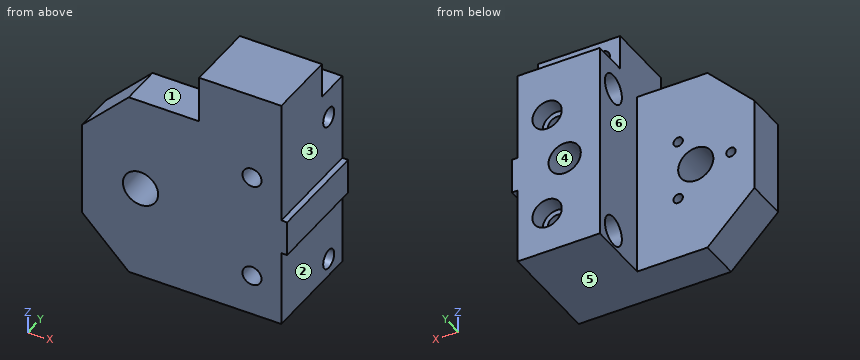
from build123d import *

# Parameters (mm, degrees)
BOSS_EXTRUDE1_DEPTH = 11.1125
BOSS_EXTRUDE2_START = -11.1125
SKETCH2_W           = 44.45
SKETCH2_H           = 127
BOSS_EXTRUDE2_DEPTH = 38.1
BOSS_EXTRUDE3_START = 26.9875
SKETCH3_W           = 44.45
SKETCH3_H           = 107.95
BOSS_EXTRUDE3_DEPTH = 19.05
BOSS_EXTRUDE4_START = -11.1125
SKETCH4_W           = 3.175
SKETCH4_H           = 19.0246
BOSS_EXTRUDE4_DEPTH = 57.15
CUT_EXTRUDE2_START  = 11.1125
SKETCH5_R           = 9.525
CUT_EXTRUDE2_DEPTH  = 131.386478852
CUT_EXTRUDE4_START  = 11.1125
SKETCH6_R           = 2.5527
CUT_EXTRUDE4_DEPTH  = 12.7
CUT_EXTRUDE6_START  = 11.1125
SKETCH7_R           = 2.5527
CUT_EXTRUDE6_DEPTH  = 12.7
CUT_EXTRUDE8_START  = 46.0375
SKETCH8_R           = 8.73125
CUT_EXTRUDE8_DEPTH  = 31.75
CUT_EXTRUDE10_START = 26.9875
SKETCH9_R           = 3.96875
CUT_EXTRUDE10_DEPTH = 19.05
CUT_EXTRUDE12_START = 46.0375
SKETCH10_R          = 5.1562
CUT_EXTRUDE12_DEPTH = 166.311478852
CUT_EXTRUDE14_START = 46.0375
SKETCH11_R          = 7.9375
CUT_EXTRUDE14_DEPTH = 9.525
CUT_EXTRUDE16_START = 31.75
SKETCH12_R          = 5.1562
CUT_EXTRUDE16_DEPTH = 88.523978852
CUT_EXTRUDE18_START = 31.75
SKETCH13_R          = 7.9375
CUT_EXTRUDE18_DEPTH = 9.525


with BuildPart() as part:
    # Sketch1 → Boss-Extrude1 (new, symmetric)
    with BuildSketch(Plane(origin=(0, 0, 0), x_dir=(1, 0, 0), z_dir=(0, 1, 0))):
        Polygon((-31.75, -25.4), (-6.35, -50.8), (31.75, -50.8), (31.75, 50.8), (-6.35, 50.8), (-31.75, 25.4), align=None)
    extrude(amount=BOSS_EXTRUDE1_DEPTH, both=True)

    # Sketch2 → Boss-Extrude2 (add)
    with BuildSketch(Plane(origin=(0, 0, 0), x_dir=(1, 0, 0), z_dir=(0, 1, 0)).offset(BOSS_EXTRUDE2_START)):
        with Locations((53.975, -12.7)):
            Rectangle(SKETCH2_W, SKETCH2_H)
    extrude(amount=BOSS_EXTRUDE2_DEPTH)

    # Sketch3 → Boss-Extrude3 (add)
    with BuildSketch(Plane(origin=(0, 0, 0), x_dir=(1, 0, 0), z_dir=(0, 1, 0)).offset(BOSS_EXTRUDE3_START)):
        with Locations((53.975, -3.175)):
            Rectangle(SKETCH3_W, SKETCH3_H)
    extrude(amount=BOSS_EXTRUDE3_DEPTH)

    # Sketch4 → Boss-Extrude4 (add)
    with BuildSketch(Plane(origin=(0, 0, 0), x_dir=(1, 0, 0), z_dir=(0, 1, 0)).offset(BOSS_EXTRUDE4_START)):
        with Locations((77.7875, 0.0127)):
            Rectangle(SKETCH4_W, SKETCH4_H)
    extrude(amount=BOSS_EXTRUDE4_DEPTH)

    # Sketch5 → Cut-Extrude2 (cut, through all)
    with BuildSketch(Plane(origin=(0, 0, 0), x_dir=(1, 0, 0), z_dir=(0, 1, 0)).offset(CUT_EXTRUDE2_START)):
        with Locations(Location((0, 0, 0), (0, 0, 270))):
            Circle(SKETCH5_R)
    extrude(amount=-CUT_EXTRUDE2_DEPTH, mode=Mode.SUBTRACT)

    # Sketch6 → Cut-Extrude4 (cut)
    with BuildSketch(Plane(origin=(0, 0, 0), x_dir=(1, 0, 0), z_dir=(0, 1, 0)).offset(CUT_EXTRUDE4_START)):
        with Locations(Location((-19.05, 0, 0), (0, 0, 270))):
            Circle(SKETCH6_R)
        with Locations(Location((9.525, -16.51, 0), (0, 0, 270))):
            Circle(SKETCH6_R)
    extrude(amount=-CUT_EXTRUDE4_DEPTH, mode=Mode.SUBTRACT)

    # Sketch7 → Cut-Extrude6 (cut)
    with BuildSketch(Plane(origin=(0, 0, 0), x_dir=(1, 0, 0), z_dir=(0, 1, 0)).offset(CUT_EXTRUDE6_START)):
        with Locations(Location((9.525, 16.51, 0), (0, 0, 270))):
            Circle(SKETCH7_R)
    extrude(amount=-CUT_EXTRUDE6_DEPTH, mode=Mode.SUBTRACT)

    # Sketch8 → Cut-Extrude8 (cut)
    with BuildSketch(Plane(origin=(0, 0, 0), x_dir=(1, 0, 0), z_dir=(0, 1, 0)).offset(CUT_EXTRUDE8_START)):
        with Locations(Location((50.8, 0, 0), (0, 0, 270))):
            Circle(SKETCH8_R)
    extrude(amount=-CUT_EXTRUDE8_DEPTH, mode=Mode.SUBTRACT)

    # Sketch9 → Cut-Extrude10 (cut)
    with BuildSketch(Plane(origin=(0, 0, 0), x_dir=(1, 0, 0), z_dir=(0, 1, 0)).offset(CUT_EXTRUDE10_START)):
        with Locations(Location((41.275, -66.675, 0), (0, 0, 270))):
            Circle(SKETCH9_R)
        with Locations(Location((66.675, -66.675, 0), (0, 0, 270))):
            Circle(SKETCH9_R)
    extrude(amount=-CUT_EXTRUDE10_DEPTH, mode=Mode.SUBTRACT)

    # Sketch10 → Cut-Extrude12 (cut, through all)
    with BuildSketch(Plane(origin=(0, 0, 0), x_dir=(1, 0, 0), z_dir=(0, 1, 0)).offset(CUT_EXTRUDE12_START)):
        with Locations(Location((60.325, -28.575, 0), (0, 0, 270))):
            Circle(SKETCH10_R)
        with Locations(Location((60.325, 28.575, 0), (0, 0, 270))):
            Circle(SKETCH10_R)
    extrude(amount=-CUT_EXTRUDE12_DEPTH, mode=Mode.SUBTRACT)

    # Sketch11 → Cut-Extrude14 (cut)
    with BuildSketch(Plane(origin=(0, 0, 0), x_dir=(1, 0, 0), z_dir=(0, 1, 0)).offset(CUT_EXTRUDE14_START)):
        with Locations(Location((60.325, -28.575, 0), (0, 0, 270))):
            Circle(SKETCH11_R)
        with Locations(Location((60.325, 28.575, 0), (0, 0, 270))):
            Circle(SKETCH11_R)
    extrude(amount=-CUT_EXTRUDE14_DEPTH, mode=Mode.SUBTRACT)

    # Sketch12 → Cut-Extrude16 (cut, through all)
    with BuildSketch(Plane(origin=(0, 0, 0), x_dir=(0, 0, -1), z_dir=(1, 0, 0)).offset(CUT_EXTRUDE16_START)):
        with Locations(Location((-41.275, 33.3375, 0), (0, 0, 180))):
            Circle(SKETCH12_R)
        with Locations(Location((41.275, 33.3375, 0), (0, 0, 180))):
            Circle(SKETCH12_R)
    extrude(amount=CUT_EXTRUDE16_DEPTH, mode=Mode.SUBTRACT)

    # Sketch13 → Cut-Extrude18 (cut)
    with BuildSketch(Plane(origin=(0, 0, 0), x_dir=(0, 0, -1), z_dir=(1, 0, 0)).offset(CUT_EXTRUDE18_START)):
        with Locations((-41.275, 33.3375)):
            Circle(SKETCH13_R)
        with Locations((41.275, 33.3375)):
            Circle(SKETCH13_R)
    extrude(amount=CUT_EXTRUDE18_DEPTH, mode=Mode.SUBTRACT)


solid = part.part
Geometry: final body of the model. Coordinates: model frame, mm. Face numbers are marked on the shaded views. A direction names the side the tool comes from. Give positions to 0.01 mm unless a question says otherwise; leave off trailing zeros. Loops run counter-clockwise (first coordinate to the right, second up) from the corner with the lowest first, then second, coordinate; pieces in that order, holes last. Notation, with made-up numbers: (-10.75, -6.5) -> (8.25, -6.5) arc R19 cw to (8.25, 9.5) -> close; hole circle Ø11 at (-4, 45.5). An arc over 180 degrees is marked (long way). Put each result on its own line as item: value.
1. Pin query (flat end, axial travel): P1, Ø12.5, axis at x = 61.5, z = 28.5, coming from the +Y side; P2, Ø7, axis at x = 41.275, z = 66.675, coming from the +Y side; P3, Ø14.5, axis at y = 33.34, z = 41.28, coming from the -X side (3 decimals). Return the tip coordinate at first contact, or that it passes through.
Taken from the geometry:
P1: stops at y = 36.51
P2: stops at y = 7.94
P3: stops at x = 41.275
2. Cut plane D-D (x = -19.05). Return the cut outline in (y, z), plus the area to 3 significant figures.
Taken from the geometry:
outline: (-11.11, -38.1) -> (11.11, -38.1) -> (11.11, -2.55) -> (-1.59, -2.55) -> (-1.59, 2.55) -> (11.11, 2.55) -> (11.11, 38.1) -> (-11.11, 38.1) -> close
area: 1,630 mm2
3. Pull-direction query (Z, two-part tool) for the marked faces 4, 5 and 6; classes: released by +Z, released by -Z, zero draft, split by the parting line, or undercut.
Taken from the geometry:
face 4: undercut
face 5: released by -Z
face 6: zero draft
4. Ray query, line 1 along X through (y, z) = (5.5, 16.51); line 2 along X through (y, z) = (-5, 0) (3 decimals); line 3 along Z through (x, y) = (66.5, 34.5). Return the intervals inside material, ascending. Write a range as [from, to].
Taken from the geometry:
line 1: x = [-31.75, 6.97], [12.08, 76.2]
line 2: x = [-31.75, -9.525], [9.525, 79.375]
line 3: z = [-50.8, -46.3], [-36.25, 36.25], [46.3, 57.15]
5. Cut plane B-B (x = 35). Count the separate pieces of the cut face and the enclosed holes in it, plus the area to 3 significant figures.
Taken from the geometry:
separate pieces: 1
enclosed holes: 2
area: 6,500 mm2
6. Set-up query: the marked faces 1, 2 and 3. Return all of +Z, -Z, +X, -X, +Y, -Y with unobstructed straight access to the full face (end or side cutting, diameter ignored); none if empty.
Taken from the geometry:
face 1: +Z, -X, +Y, -Y
face 2: -Z, +X, +Y, -Y
face 3: +Z, +X, +Y, -Y
